from build123d import *

# Parameters (mm, degrees)
BOSS_EXTRUDE1_DEPTH = 10.16
SKETCH3_W           = 10.16
SKETCH3_H           = 5.08
BOSS_EXTRUDE2_DEPTH = 16.51
SKETCH4_W           = 10.16
SKETCH4_H           = 5.08
BOSS_EXTRUDE3_DEPTH = 16.51
BOSS_EXTRUDE4_DEPTH = 5.08


with BuildPart() as part:
    # Sketch1 → Boss-Extrude1 (new body)
    with BuildSketch(Plane(origin=(0, 0, 0), x_dir=(1, 0, 0), z_dir=(0, 1, 0))):
        with BuildLine():
            Line((0, -32.004), (0, -35.179))
            ThreePointArc((0, -35.179), (-35.156038364, -1.270829481), (-2.54, 35.087183429))
            Line((-2.54, 35.087183429), (-2.54, 31.903047127))
            ThreePointArc((-2.54, 31.903047127), (-31.978751823, -1.271002703), (0, -32.004))
        make_face()
    extrude(amount=BOSS_EXTRUDE1_DEPTH)

    # Sketch3 → Boss-Extrude2 (add)
    with BuildSketch(Plane(origin=(0, 0, 32.004), x_dir=(0, -1, 0), z_dir=(0, 0, -1))):
        with Locations((-5.08, 2.54)):
            Rectangle(SKETCH3_W, SKETCH3_H)
    extrude(amount=-BOSS_EXTRUDE2_DEPTH)

    # Sketch4 → Boss-Extrude3 (add)
    with BuildSketch(Plane(origin=(0, 0, -32.004), x_dir=(0, -1, 0), z_dir=(0, 0, 1))):
        with Locations((-5.08, -5.08)):
            Rectangle(SKETCH4_W, SKETCH4_H)
    extrude(amount=-BOSS_EXTRUDE3_DEPTH)

    # Sketch5 → Boss-Extrude4 (add)
    with BuildSketch(Plane(origin=(0, 10.16, 0), x_dir=(1, 0, 0), z_dir=(0, 1, 0))):
        Polygon((-22.630245425, -22.630245425), (-34.304578382, -34.304578382), (-41.488783279, -27.120373486), (-29.814450322, -15.446040528), align=None)
    extrude(amount=-BOSS_EXTRUDE4_DEPTH)


solid = part.part
Verification items for the finished model (mm, model axes). A direction names the side the tool comes from. Give positions to 0.01 mm unless a question says otherwise; leave off trailing zeros. Loops run counter-clockwise (first coordinate to the right, second up) from the corner with the lowest first, then second, coordinate; pieces in that order, holes last. Notation, with made-up numbers: (39, -33.5) - (60, -33.5) arc R32 cw to (60, 0.5) - close; hole circle Ø8 at (-38, -8.5). An arc over 180 degrees is marked (long way). Write item = value, one per line. Start each with the question number.
Q1. Cross-section at C-C, the plane y = 6.75. Enter the section's corners in (x, z).
Q2. Depth check by flat-ended pin: P1, Ø13.5, axis at x = -35, z = 25.5, coming from the -Y side; P2, Ø3, axis at y = 7, z = -39, coming from the -X side; P3, Ø6, axis at y = 2.5, z = 8, coming from the +X side; P4, Ø10, axis at x = -18.5, z = -16.5, coming from the -Y side. Enter the tip coordinate at first touch or a pass-through.
Q3. Thickness scan on line 1 (X direction, y = 4, z = -42.5); line 2 (Z direction, x = -23, y = 2.5); line 3 (X direction, y = 8.5, z = 25). Record the ranges inside material, lowest first.
Q4. Tool access check on faces 4 (the face through (-7.62, 5, -41)), 5 (the face through (-5.08, 5, 42)), 6 (the face through (-33, 5.08, 25)). Record the directions out of +Z, -Z, +X, -X, +Y, -Y that give a thin tool (end or side, any length) a straight path to the whole face; none if there is none.
Q5. Cross-section at D-D, the plane z = 38.5. Enter the section's corners in (x, y).
Q6. Mould release check, pull along Z, two halves, no side actions. Record for faces 1 (the face through (-36.32, 7.66, 21.95)), 2 (the face through (-5, 5, -48.514)), 3 (the face through (-2.54, 5, -40)): released by +Z, released by -Z, zero draft, split by the parting line, or undercut.
Q7. Cross-section at B-B, the plane x = -21. Enter the section's corners in (y, z), and give its area (3 significant figures).
Q8. Cross-section at A-A, the plane y = 2.25. Enter the section's corners in (x, z).
Answer key:
q1.outline = (-41.49, 27.12) - (-31, 16.63) arc R35.18 ccw to (-7.62, -34.34) - (-7.62, -48.51) - (-2.54, -48.51) - (-2.54, -31.9) arc R32 cw to (0, 32) - (0, 48.51) - (-5.08, 48.51) - (-5.08, 34.81) arc R35.18 ccw to (-24.88, 24.88) - (-34.3, 34.3) - close
q2.P1 = 5.08
q2.P2 = -7.62
q2.P3 = -30.05
q2.P4 = through
q3.line_1 = -7.62 to -2.54
q3.line_2 = -26.62 to -22.25, 22.25 to 26.62
q3.line_3 = -39.37 to -25, -24.75 to -19.98
q4.face_4 = -Z, -X, +Y, -Y
q4.face_5 = +Z, -X, +Y, -Y
q4.face_6 = +Z, -X, -Y
q5.outline = (-5.08, 0) - (0, 0) - (0, 10.16) - (-5.08, 10.16) - close
q6.face_1 = undercut
q6.face_2 = released by -Z
q6.face_3 = zero draft
q7.outline = (0, -28.22) - (10.16, -28.22) - (10.16, -24.15) - (0, -24.15) - close; (0, 24.15) - (10.16, 24.15) - (10.16, 28.22) - (0, 28.22) - close
q7.area = 82.8 mm^2
q8.outline = (-7.62, -48.51) - (-2.54, -48.51) - (-2.54, -31.9) arc R32 cw to (0, 32) - (0, 48.51) - (-5.08, 48.51) - (-5.08, 34.81) arc R35.18 ccw to (-7.62, -34.34) - close
